The figure shows three views and two pictorial views of one solid part (mm, origin at its lowest corner). Answer the questions. Round coordinates to 2 decimals unless told otherwise and drop trailing zeros. Write each loop counter-clockwise with the first axis right and the second up, starting at its lowest first coordinate (ties: lowest second). Pieces come first, ordered by that corner, then holes.
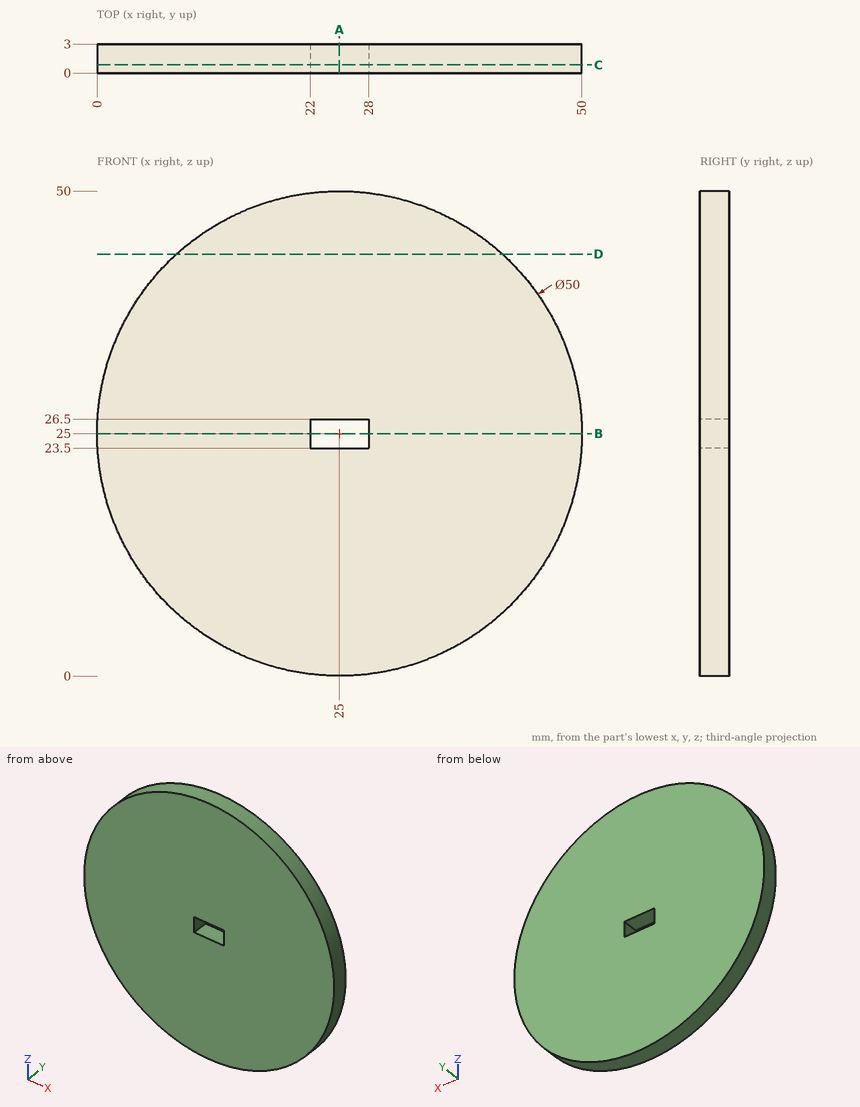
Q1. Section B-B (z = 25) is taken. Determine the outline of the cut face in (x, y), then the cut area to 3 significant figures.
Verdict:
outline: (0, 0) - (22, 0) - (22, 3) - (0, 3) - close; (28, 0) - (50, 0) - (50, 3) - (28, 3) - close
area: 132 mm2
Q2. Section A-A (x = 25) is taken. Determine the outline of the cut face in (y, z).
Verdict:
outline: (0, 0) - (3, 0) - (3, 23.5) - (0, 23.5) - close; (0, 26.5) - (3, 26.5) - (3, 50) - (0, 50) - close
Q3. Section C-C (y = 0.85) is taken. Determine the outline of the cut face in (x, z).
Verdict:
outline: circle Ø50 at (25, 25); hole (22, 23.5) - (28, 23.5) - (28, 26.5) - (22, 26.5) - close
Q4. Section D-D (z = 43.5) is taken. Determine the outline of the cut face in (x, y).
Verdict:
outline: (8.18, 0) - (41.82, 0) - (41.82, 3) - (8.18, 3) - close
Q5. Flat-ended cylindrical pins translate along their axes: pin 1 Ø1.5 at (x, y) = (23.5, 1) entering from +Z; pin 2 Ø1 at (y, z) = (2.5, 28) entering from +X; pin 3 Ø1.5 at (x, y) = (25, 2) entering from -Z. Find the tip coordinate at first contact, or state that the pin passes through.
Verdict:
pin 1: stops at z = 49.99
pin 2: stops at x = 49.87
pin 3: stops at z = 0
Q6. Straight lines are drawn through the part: probe 1 along Z at (x, y) = (25.5, 2.1) (3 decimals); probe 2 along Z at (x, y) = (22.5, 1.5); probe 3 along X at (y, z) = (0.7, 30.5). For each, find the intervals that lie inside material, in ascending order.
Verdict:
probe 1: z = 0.005 to 23.5, 26.5 to 49.995
probe 2: z = 0.13 to 23.5, 26.5 to 49.87
probe 3: x = 0.61 to 49.39
